Geometry check sheet. Reference: the model listing, model coordinates, mm. A direction names the side the tool comes from. Coordinates: 2 decimals unless noted, no trailing zeros. Order: outer loops, then holes, each group sorted by start corner. A loop starts at its lowest first (then second) coordinate and runs counter-clockwise, first axis right, second up. Notation, with made-up numbers: M 51,-15 L 68,-15 A33 cw 68,20 Z; hole C -25.75,-16 d1. An arc over 180 degrees is marked long. One line per item, written item: value. Start each with the question number.
1) Sectioned sample at C-C, the plane z = -4. Enter the section's corners in (x, y).
2) Sectioned sample at A-A, the plane y = 5. Enter the section's corners in (x, z), then the cut area to 3 significant figures.
3) Access from +Z, -Z, +X, -X, +Y, -Y to the whole of each face (thin tool, end or side, straight path). Record for faces 1 (the cylindrical face through (0.14, 0.54, 19.48)), 2 (the flat face through (0, 1.5, 0)), 3 (the cylindrical face through (-0.112, 37.648, 19.24)), 4 (the cylindrical face through (6.96, 28.34, -19.26)), 5 (the cylindrical face through (-9.715, 34.899, -19.26)).
4) Draft check along X on faces 6 (the cylindrical face through (-0.1, 28.7, -19.2)), 7 (the flat face through (-8, 35.2, -19)), 8 (the cylindrical face through (-8.71, 28.974, -19.26)), 9 (the cylindrical face through (9.699, 34.915, -19.26)). Enter one of: pulls with the +X half, pulls with the -X half, needs draft (parallel to the pull), parting line crosses it, or undercut.
5) Thickness scan on L1, parallel to X at y = 14.98, z = -19; L2, parallel to X at y = 0.7, z = 9.5; L3, parallel to X at y = 35.1, z = 19.45. Record the ranges inside material, lowest first. Write a range as from..to.
6) Go/stop test with flat-tipped pins: P1, Ø4, axis at x = -7, z = -4.5, coming from the +Y side; P2, Ø1.3, axis at x = -7, y = 14.98, coming from the -Z side; P3, Ø12, axis at y = 35, z = -11, coming from the -X side; P4, Ø1.2, axis at x = 7.5, z = -19.5, coming from the +Y side. Record where each tip stops, or that it passes through.
7) Sectioned sample at D-D, the plane x = -4.25. Enter the section's corners in (y, z).
8) Sectioned sample at B-B, the plane x = 0. Enter the section's corners in (y, z).
Autodesk Inventor part; units mm, degrees
ref_plane "YZ Plane" through (0, 0, 0) normal (1, 0, 0) x (0, 1, 0)
ref_plane "XZ Plane" through (0, 0, 0) normal (0, 1, 0) x (-1, 0, 0)
ref_plane "XY Plane" through (0, 0, 0) normal (0, 0, 1) x (1, 0, 0)
sketch "Sketch1" plane through (0, 0, 0) normal (0, 1, 0) x (-1, 0, 0)
  line L0 (10, -18.5) -> (-10, -18.5)
  line L1 (-10, -18.5) -> (-10, 18.5)
  line L2 (-10, 18.5) -> (10, 18.5)
  line L3 (10, 18.5) -> (10, -18.5)
  point P0 (0, 0)
  dimension "d0" = 20
  dimension "d1" = 37
  dimension "d2" = 18.5
  dimension "d3" = 10
extrude "Plate1" add sketch "Sketch1" along normal blind 1.5
sketch "Sketch2" plane through (-10, 0, -20) normal (0, 0, 1) x (1, 0, 0)
  line L0 (20, 0) -> (0, 0)
  line L1 (0, 0) -> (0, 45.1)
  line L2 (0, 45.1) -> (20, 45.1)
  line L3 (20, 45.1) -> (20, 0)
edge flange "Flange1" height 45.1 angle 90 thickness 1.5 bend radius 0.31 thickness toward (0, 0, 1) relief tear relief width 1.5 relief depth 0.75 edges at (0, 1.5, -18.5) wall of the first edge with corners at (10, 0, -20) (-10, 0, -20) (-10, 45.1, -20) (10, 45.1, -20)
bend "Bend1"
corner "Corner1"
sketch "Sketch3" plane through (10, 0, 20) normal (0, 0, -1) x (-1, 0, 0)
  line L0 (20, 0) -> (0, 0)
  line L1 (0, 0) -> (0, 45.1)
  line L2 (0, 45.1) -> (20, 45.1)
  line L3 (20, 45.1) -> (20, 0)
edge flange "Flange2" height 45.1 angle 90 thickness 1.5 bend radius 0.31 thickness toward (0, 0, -1) relief tear relief width 1.5 relief depth 0.75 edges at (0, 1.5, 18.5) wall of the first edge with corners at (-10, 0, 20) (10, 0, 20) (10, 45.1, 20) (-10, 45.1, 20)
bend "Bend2"
corner "Corner2"
sketch "Sketch4" plane through (-10, 45.1, 20) normal (0, 0, 1) x (1, 0, 0)
  circle A0 centre (10, -10) radius 10
  line L0 (0, 0) -> (20, 0)
  line L1 (0, 0) -> (20, 0)
  line L2 (20, 0) -> (20, -10)
  line L3 (20, -10) -> (0, -10)
  line L4 (0, -10) -> (0, 0)
  line L5 (0, -43.29) -> (0, 0)
  point P0 (10, -45.1)
  point P1 (10, -10)
  point P2 (20, 0)
  point P3 (10, 0)
  point P4 (0, -10)
  point P5 (8.5893, 0)
  point P6 (0, -10)
  dimension "d26" = 20
  dimension "d25" = 10
  dimension "d27" = 10
  dimension "d28" = 10
extrude "Extrusion1" cut sketch "Sketch4" against normal blind 10 contours L4 L0 A0 | A0 L0 L2
sketch "Sketch5" plane through (10, 45.1, -20) normal (0, 0, -1) x (-1, 0, 0)
  arc A0 (20, -10) -> (0, -10) centre (10, -10) ccw
  point P0 (10, -45.1)
hole "Hole1" at (0, 35.1, -20) direction (0, 0, 1) diameter 12.8 depth 1.5
sketch "Sketch6" plane through (10, 45.1, -20) normal (0, 0, -1) x (-1, 0, 0)
  circle A0 centre (10, -10) radius 6.4
  line L0 (0, 0) -> (20, 0)
  line L1 (0, -43.29) -> (0, 0)
  line L2 (24, 0) -> (-4, 0)
  line L3 (-4, 0) -> (-4, -9.9)
  line L4 (-4, -9.9) -> (24, -9.9)
  line L5 (24, -9.9) -> (24, 0)
  point P0 (10, -45.1)
  point P1 (20, 0)
  point P2 (6.005, 0)
  point P3 (13.995, 0)
  dimension "d38" = 9.9
  dimension "d39" = 4
  dimension "d40" = 28
extrude "Extrusion2" cut sketch "Sketch6" against normal blind 10 contours L4 A0 | A0 L4 L1 L0 L2 L5 | L4 L3 L2 L1 picked at (9.1972, -6.4205)
fillet "Fillet1" radius 1 2 edges at (-10, 35.2, -19.25) (10, 35.2, -19.25)
sketch "Sketch7" plane through (-10, 1.81, 20) normal (0, 0, 1) x (1, 0, 0)
  arc A0 (20, 33.29) -> (0, 33.29) centre (10, 33.29) ccw
  point P0 (10, -1.81)
hole "Hole2" at (0, 35.1, 20) direction (0, 0, -1) diameter 5.1 depth 1.5
sketch "Sketch8" plane through (0, 0, 0) normal (0, -1, 0) x (1, 0, 0)
  line L0 (2.55, 18.5) -> (-2.55, 18.5)
  line L1 (-10, 18.5) -> (10, 18.5)
  line L2 (10, 18.5) -> (-10, 18.5)
  line L3 (10, 18.19) -> (-10, 18.19)
  line L4 (-10, -18.19) -> (-10, 18.19)
  line L5 (-10, -18.19) -> (10, -18.19)
  line L6 (10, 18.19) -> (10, -18.19)
  point P0 (0, 0)
  point P1 (7, 9.5)
  point P2 (7, -4.5)
  point P3 (-7, 9.5)
  point P4 (-7, -4.5)
  dimension "d51" = 9
  dimension "d52" = 3
  dimension "d55" = 14
  dimension "d58" = 14
hole "Hole3" at (7, 0, 9.5) at (7, 0, -4.5) at (-7, 0, 9.5) at (-7, 0, -4.5) direction (0, 1, 0) diameter 3 depth 1.5
sketch "Sketch11" plane through (-10, 1.81, -18.5) normal (0, 0, 1) x (1, 0, 0)
  circle A0 centre (18, 26.39) radius 0.7835
  circle A1 centre (2, 26.39) radius 0.7835
  circle A2 centre (17, 13.17) radius 0.7835
  circle A3 centre (3, 13.17) radius 0.7835
  circle A4 centre (10, 5.87) radius 0.7835
  point P0 (10, -1.81)
hole "Hole6" at (-8, 28.2, -18.5) at (-7, 14.98, -18.5) at (0, 7.68, -18.5) at (7, 14.98, -18.5) at (8, 28.2, -18.5) direction (0, 0, -1) diameter 2.1 depth 1.5
equation "\"d36\" = Thickness"
equation "\"d49\" = Thickness"
equation "\"d66\" = Thickness"
equation "\"d87\" = Thickness"
equation "\"d4\" = Thickness"
equation "\"d5\" = BendReliefWidth"
equation "\"d6\" = BendReliefDepth"
equation "\"d7\" = MinimumRemnant"
equation "\"d8\" = TransitionRadius"
equation "\"d11\" = BendRadius"
equation "\"d12\" = CornerReliefSize"
equation "\"d13\" = GapSize"
equation "\"d14\" = JacobiRadiusSize"
equation "\"d15\" = BendReliefWidth"
equation "\"d16\" = BendReliefDepth"
equation "\"d17\" = MinimumRemnant"
equation "\"d18\" = TransitionRadius"
equation "\"d21\" = BendRadius"
equation "\"d22\" = CornerReliefSize"
equation "\"d23\" = GapSize"
equation "\"d24\" = JacobiRadiusSize"
equation "\"BendReliefWidth\" = Thickness"
equation "\"BendReliefDepth\" = 0.5 * Thickness"
equation "\"CornerReliefSize\" = 4 * Thickness"
equation "\"MinimumRemnant\" = 2 * Thickness"
equation "\"TransitionRadius\" = BendRadius"
equation "\"JacobiRadiusSize\" = BendRadius"
equation "\"GapSize\" = Thickness"
properties part number "axis_9_bottom_frame" material "Aluminum 6061-AHC"
Final values:
1. outline: M -10,0 L -8.41,0 L -8.41,1.5 L -10,1.5 Z; M -5.59,0 L 5.59,0 L 5.59,1.5 L -5.59,1.5 Z; M 8.41,0 L 10,0 L 10,1.5 L 8.41,1.5 Z
2. outline: M -10,-20 L 10,-20 L 10,-18.5 L -10,-18.5 Z; M -10,18.5 L 10,18.5 L 10,20 L -10,20 Z
2. area: 60.0 mm^2
3. face 1: +Z, +X, -X, -Y
3. face 2: +X, -X, +Y
3. face 3: +Z, -Z
3. face 4: -Z
3. face 5: -Z, -X, +Y
4. face 6: undercut
4. face 7: needs draft
4. face 8: undercut
4. face 9: pulls with the +X half
5. L1: x = -10..-8.05, -5.95..5.95, 8.05..10
5. L2: x = -10..-8.5, -5.5..5.5, 8.5..10
5. L3: x = -10..-2.55, 2.55..10
6. P1: stops at y = 1.5
6. P2: stops at z = 18.5
6. P3: passes through
6. P4: stops at y = 35.2
7. outline: M 0,-18.19 A1.81 ccw 1.81,-20 L 30.31,-20 L 30.31,-18.5 L 1.81,-18.5 A0.31 cw 1.5,-18.19 L 1.5,18.19 A0.31 cw 1.81,18.5 L 44.15,18.5 L 44.15,20 L 1.81,20 A1.81 ccw 0,18.19 Z
8. outline: M 0,-18.19 A1.81 ccw 1.81,-20 L 6.63,-20 L 6.63,-18.5 L 1.81,-18.5 A0.31 cw 1.5,-18.19 L 1.5,18.19 A0.31 cw 1.81,18.5 L 32.55,18.5 L 32.55,20 L 1.81,20 A1.81 ccw 0,18.19 Z; M 8.73,-20 L 28.7,-20 L 28.7,-18.5 L 8.73,-18.5 Z; M 37.65,18.5 L 45.1,18.5 L 45.1,20 L 37.65,20 Z
